```python
from build123d import *

# Parameters (mm, degrees)
F0_W     = 50.8
F0_H     = 50.8
F0_R     = 11.596752
F1_DEPTH = 50.8
F2_W     = 21.541153
F2_H     = 25.131345
F3_DEPTH = 25.4
F4_W     = 21.284714
F4_H     = 23.849137
F5_DEPTH = 12.7


with BuildPart() as f1:
    # F0 (on Front) → F1 (new body)
    with BuildSketch(Plane.XZ):
        with Locations((-25.4, 25.4)):
            Rectangle(F0_W, F0_H)
        with Locations((-25.4, 25.4)):
            Circle(F0_R, mode=Mode.SUBTRACT)
    extrude(amount=F1_DEPTH)

    # F2 (on face) → F3 (join)
    with BuildSketch(Plane.YZ):
        with Locations((-24.105576, 28.336875)):
            Rectangle(F2_W, F2_H)
    extrude(amount=F3_DEPTH)

    # F4 (on face) → F5 (join)
    with BuildSketch(Plane(origin=(-50.8, 0, 0), x_dir=(0, -1, 0), z_dir=(-1, 0, 0))):
        with Locations((26.541781, 25.644231)):
            Rectangle(F4_W, F4_H)
    extrude(amount=F5_DEPTH)


solid = f1.part
```
The model under review builds one solid part; all positions refer to its coordinate system, in mm. A direction names the side the tool comes from. Round coordinates to 2 decimals unless told otherwise and drop trailing zeros. Loops run counter-clockwise (first coordinate to the right, second up) from the corner with the lowest first, then second, coordinate; pieces in that order, holes last. Notation, with made-up numbers: (55, 87) - (86, 87) arc R26 cw to (86, 107) - close; hole circle Ø9 at (0, 89.5). An arc over 180 degrees is marked (long way). Use a Markdown table: item, result. Add a question column.
Q1. The part is to be moulded in two halves that separate along Z. For faces 6 (the face through (-31, -50.8, 37)), 7 (the face through (-57, -26, 13.72)), 8 (the face through (-20.05, -25.04, 15.11)), say which applies: pulls with the +Z half, pulls with the -Z half, needs draft (parallel to the pull), parting line crosses it, or undercut.
Q2. Add section B-B (y = -21.5). State the section outline as (x, z) points, plus the area to 3 significant figures.
Q3. For probe 1 along Z at (x, y) = (-25.4, -40); probe 2 along X at (y, z) = (-20, 25); probe 3 along X at (y, z) = (-28, 47.5), list the stretches that pass through material, from the lowest coordinate up.
Q4. Machinability: for faces 1 (the face through (-57, -26, 37.569)), 2 (the face through (13, -24, 15.771)), 3 (the face through (13, -34.876, 28)), 4 (the face through (-57, -15.899, 25)), 5 (the face through (13, -13.335, 28)), which of the approach directions +Z, -Z, +X, -X, +Y, -Y give a long, thin tool a straight path to every point of the face, cutting with its end or side? Answer none if there is none.
Q5. Add section D-D (z = 34.5). State the section outline as (x, y) points (1 decimal).
Q6. Add section C-C (x = -25.4). State the section outline as (y, z) points, plus the area to 3 significant figures.
Q7. Add section A-A (z = 25.4). State the section outline as (x, y) points (3 decimals).
Q8. Insertion check: pin 1 Ø4 at (x, z) = (-58.5, 28.5) entering from -Y; pin 2 Ø10 at (x, y) = (-60, -26.5) entering from +Z; pin 3 Ø23.5 at (x, y) = (13, -20.5) entering from -Z; pin 4 Ø3 at (x, z) = (-30, 18) entering from +Y (1 decimal). Each pin has a flat end and moves straight along its axis. Give the tip position at first contact, or say it passes through.
Worked answers:
| question | item | result |
|---|---|---|
| 1 | face 6 | needs draft |
| 1 | face 7 | pulls with the -Z half |
| 1 | face 8 | undercut |
| 2 | outline | (-63.5, 13.72) - (-50.8, 13.72) - (-50.8, 0) - (0, 0) - (0, 15.77) - (25.4, 15.77) - (25.4, 40.9) - (0, 40.9) - (0, 50.8) - (-50.8, 50.8) - (-50.8, 37.57) - (-63.5, 37.57) - close; hole circle Ø23.19 at (-25.4, 25.4) |
| 2 | area | 3,100 mm² |
| 3 | probe 1 | 0 to 13.8, 37 to 50.8 |
| 3 | probe 2 | -63.5 to -36.99, -13.81 to 25.4 |
| 3 | probe 3 | -50.8 to 0 |
| 4 | face 1 | +Z, -X, +Y, -Y |
| 4 | face 2 | -Z, +X, +Y, -Y |
| 4 | face 3 | +Z, -Z, +X, -Y |
| 4 | face 4 | +Z, -Z, -X, +Y |
| 4 | face 5 | +Z, -Z, +X, +Y |
| 5 | outline | (-63.5, -37.2) - (-50.8, -37.2) - (-50.8, -50.8) - (-32.6, -50.8) - (-32.6, 0) - (-50.8, 0) - (-50.8, -15.9) - (-63.5, -15.9) - close; (-18.2, -50.8) - (0, -50.8) - (0, -34.9) - (25.4, -34.9) - (25.4, -13.3) - (0, -13.3) - (0, 0) - (-18.2, 0) - close |
| 6 | outline | (-50.8, 0) - (0, 0) - (0, 13.8) - (-50.8, 13.8) - close; (-50.8, 37) - (0, 37) - (0, 50.8) - (-50.8, 50.8) - close |
| 6 | area | 1,400 mm² |
| 7 | outline | (-63.5, -37.184) - (-50.8, -37.184) - (-50.8, -50.8) - (-36.997, -50.8) - (-36.997, 0) - (-50.8, 0) - (-50.8, -15.899) - (-63.5, -15.899) - close; (-13.803, -50.8) - (0, -50.8) - (0, -34.876) - (25.4, -34.876) - (25.4, -13.335) - (0, -13.335) - (0, 0) - (-13.803, 0) - close |
| 8 | pin 1 | y = -37.18 |
| 8 | pin 2 | z = 37.57 |
| 8 | pin 3 | z = 15.77 |
| 8 | pin 4 | through |
